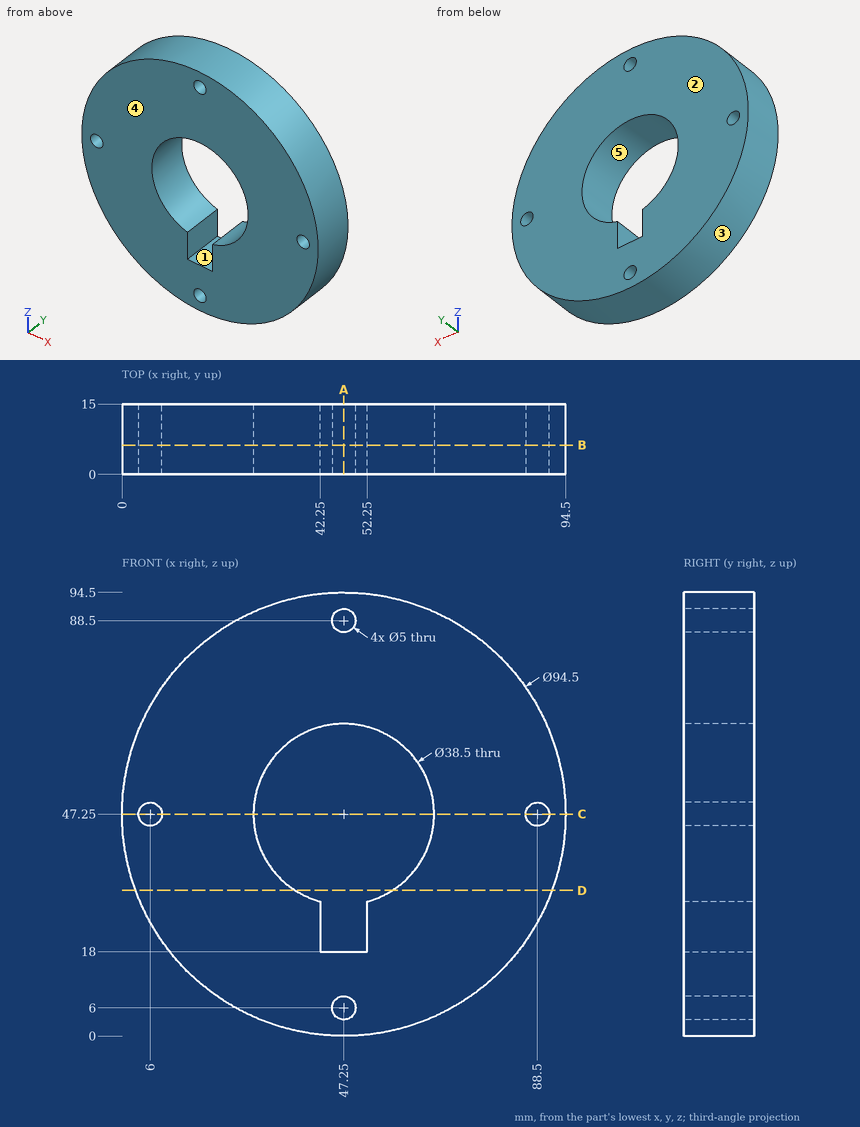
Could you check a few things on this drawing? It's one solid part, dimensions in mm from its lowest x, y, z. A direction names the side the tool comes from. Give positions to 0.01 mm unless a question says otherwise; leave off trailing zeros. Order: outer loops, then holes, each group sorted by start corner. A loop starts at its lowest first (then second) coordinate and runs counter-clockwise, first axis right, second up. Notation, with made-up numbers: M 73,-0.75 L 88,-0.75 A20 cw 88,36.25 Z; hole C 81,71 d7. An arc over 180 degrees is marked long. Use one line per item in the form item = value. Start each with the question number.
Item 1: If we section it at B-B (y = 6.25): Write out the boundary of the cut face in (x, z).
Item 2: If I drill on line 1 along X through (y, z) = (9.75, 47.25); line 2 along X through (y, z) = (10.25, 59); line 3 along X through (y, z) = (11.5, 28), over which ranges is the centre line in solid material (lowest first)?
Item 3: If we section it at A-A (x = 47.25): Write out the boundary of the cut face in (y, z).
Item 4: For the marked faces 1 and 2, which set-ups out of +Z, -Z, +X, -X, +Y, -Y let a thin tool reach every point of the face, with its end or its side?
Item 5: If we section it at C-C (z = 47.25): Write out the boundary of the cut face in (x, y), then the cut area to 3 significant figures.
Item 6: Will these pins go through, and if not, where does the flat tip stop? pin 1 Ø4 at (y, z) = (9, 52) entering from -X; pin 2 Ø2 at (x, y) = (69.5, 6.5) entering from -Z; pin 3 Ø3 at (x, y) = (49.5, 6) entering from +Z.
Item 7: If we section it at D-D (z = 31): Write out the boundary of the cut face in (x, y).
Item 8: We'd pull the mould along X, two halves only. Please class the marked faces 3, 4 and 5: +X half, -X half, draft (parallel to the pull), parting line (faces both ways), or undercut.
Outcome:
q1.outline = C 47.25,47.25 d94.5; hole C 6,47.25 d5; hole M 42.25,18 L 52.25,18 L 52.25,28.66 A19.25 ccw long 42.25,28.66 Z; hole C 47.25,6 d5; hole C 47.25,88.5 d5; hole C 88.5,47.25 d5
q2.line_1 = 0 to 3.5, 8.5 to 28, 66.5 to 86, 91 to 94.5
q2.line_2 = 1.48 to 32, 62.5 to 93.02
q2.line_3 = 4.1 to 42.25, 52.25 to 90.4
q3.outline = M 0,0 L 15,0 L 15,3.5 L 0,3.5 Z; M 0,8.5 L 15,8.5 L 15,18 L 0,18 Z; M 0,66.5 L 15,66.5 L 15,86 L 0,86 Z; M 0,91 L 15,91 L 15,94.5 L 0,94.5 Z
q4.face_1 = +Y, -Y
q4.face_2 = +Z, -Z, +X, -X, +Y
q5.outline = M 0,0 L 3.5,0 L 3.5,15 L 0,15 Z; M 8.5,0 L 28,0 L 28,15 L 8.5,15 Z; M 66.5,0 L 86,0 L 86,15 L 66.5,15 Z; M 91,0 L 94.5,0 L 94.5,15 L 91,15 Z
q5.area = 690 mm2
q6.pin_1 = 0.08
q6.pin_2 = 5.05
q6.pin_3 = 94.49
q7.outline = M 2.88,0 L 36.93,0 L 36.93,15 L 2.88,15 Z; M 57.57,0 L 91.62,0 L 91.62,15 L 57.57,15 Z
q8.face_3 = parting line
q8.face_4 = draft
q8.face_5 = undercut
